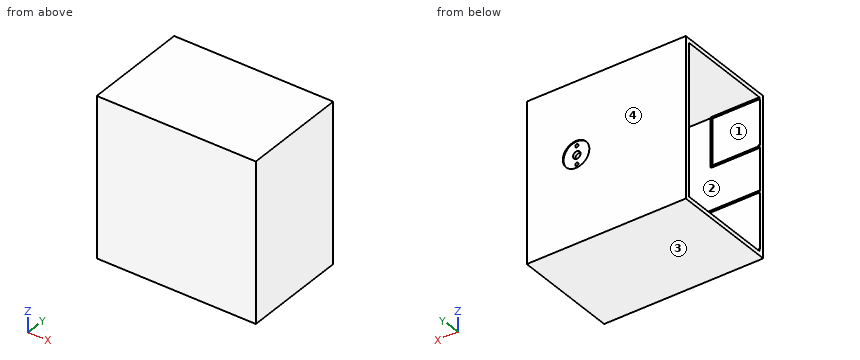
Autodesk Inventor part; units mm, degrees
ref_plane "YZ Plane" through (0, 0, 0) normal (1, 0, 0) x (0, 1, 0)
ref_plane "XZ Plane" through (0, 0, 0) normal (0, 1, 0) x (-1, 0, 0)
ref_plane "XY Plane" through (0, 0, 0) normal (0, 0, 1) x (1, 0, 0)
sketch "Boceto1" plane through (0, 0, 0) normal (0, 1, 0) x (-1, 0, 0)
  point P0 (0, 0)
extrude "Extrusión1" [suppressed]
feature "Vaciado1" [suppressed]
sketch "Boceto2" plane through (0, 70, 0) normal (0, 1, 0) x (1, 0, 0)
  line L0 (-5, 5) -> (-5, 145)
  line L1 (-145, 145) -> (-145, 5)
  line L2 (-145, 5) -> (-5, 5)
  line L3 (-5, 145) -> (-145, 145)
  line L4 (-150, 0) -> (0, 0)
  circle A0 centre (-46.4922, 78) radius 12.5
  circle A1 centre (-46.4922, 78) radius 13.5
hole "Agujero1" [suppressed]
sketch "Boceto3" plane through (0, 70, 0) normal (0, 1, 0) x (1, 0, 0)
  point P0 (0, 0)
sketch "Boceto4" plane through (0, 0, 0) normal (0, 1, 0) x (-1, 0, 0)
  point P0 (0, 0)
extrude "Extrusión2" [suppressed]
feature "Vaciado2" [suppressed]
sketch "Boceto5" plane through (0, 100, 0) normal (0, 1, 0) x (1, 0, 0)
  line L0 (0, 0) -> (0, 150)
  circle A0 centre (-46.5, 67.5) radius 14.5
extrude "Extrusión3" [suppressed]
sketch "Boceto6" plane through (0, 100, 0) normal (0, 1, 0) x (1, 0, 0)
  circle A0 centre (-46.5, 67.5) radius 12.5
extrude "Extrusión4" [suppressed]
sketch "Boceto7" plane through (-46.5, 31, -67.5) normal (0, -1, 0) x (1, 0, 0)
  point P0 (46.5, 67.5)
sketch "Boceto8" plane through (-46.5, 33, -67.5) normal (0, 1, 0) x (1, 0, 0)
  point P0 (46.5, -67.5)
sketch "Boceto9" plane through (0, 100, 0) normal (0, 1, 0) x (1, 0, 0)
  point P0 (0, 0)
sketch "Boceto10" plane through (0, 0, 0) normal (0, 1, 0) x (-1, 0, 0)
  line L0 (0, 0) -> (0, -150)
  line L1 (0, -150) -> (150, -150)
  line L2 (150, -150) -> (150, 0)
  line L3 (150, 0) -> (0, 0)
extrude "Extrusión5" add sketch "Boceto10" along normal blind 100
shell "Vaciado3" thickness 3 removed faces 1 at (-150, 33.3333, -100)
sketch "Boceto11" plane through (0, 100, 0) normal (0, 1, 0) x (1, 0, 0)
  line L0 (-150, 0) -> (0, 0)
  line L1 (0, 0) -> (0, 150)
  circle A0 centre (-46.5, 67.5) radius 12.5002
extrude "Extrusión6" add sketch "Boceto11" against normal blind 4
sketch "Boceto12" plane through (0, 100, 0) normal (0, 1, 0) x (1, 0, 0)
  circle A0 centre (-46.5, 67.5) radius 12.5
  point P0 (0, 0)
extrude "Extrusión7" cut sketch "Boceto12" against normal blind 1
sketch "Boceto13" plane through (0, 100, 0) normal (0, 1, 0) x (1, 0, 0)
  point P0 (0, 0)
sketch "Boceto14" plane through (-46.5, 96, -67.5) normal (0, -1, 0) x (1, 0, 0)
  circle A0 centre (0, 0) radius 3.5
  point P0 (46.5, 67.5)
extrude "Extrusión8" cut sketch "Boceto14" against normal blind 3
sketch "Boceto15" plane through (-46.5, 99, -67.5) normal (0, 1, 0) x (1, 0, 0)
  circle A0 centre (0, -8.5) radius 1.5
  circle A1 centre (0, 8.5) radius 1.5
  point P0 (46.5, -67.5)
extrude "Extrusión9" cut sketch "Boceto15" against normal blind 3
sketch "Boceto16" plane through (-150, 0, -150) normal (-1, 0, 0) x (0, 0, 1)
  line L0 (3, 97) -> (147, 97)
  line L1 (4, 96) -> (146, 96)
  line L2 (147, 3) -> (3, 3)
  line L3 (4, 4) -> (4, 96)
  line L4 (146, 4) -> (4, 4)
  line L5 (146, 96) -> (146, 4)
  line L6 (3, 97) -> (147, 97)
  line L7 (147, 3) -> (147, 97)
  line L8 (147, 3) -> (3, 3)
  line L9 (3, 3) -> (3, 97)
  line L10 (3, 97) -> (3, 3)
  line L11 (147, 97) -> (147, 3)
  point P0 (150, 0)
sketch "Boceto17" plane through (-150, 3, -147) normal (0, 0, 1) x (1, 0, 0)
  point P0 (150, -3)
extrude "Extrusión10" add sketch "Boceto16" against normal blind 148
sketch "Boceto18" plane through (-46.5, 97, -67.5) normal (0, 1, 0) x (1, 0, 0)
  circle A0 centre (0, 0) radius 3.5
  point P0 (46.5, -67.5)
extrude "Extrusión11" cut sketch "Boceto18" against normal blind 1
sketch "Boceto19" plane through (-150, 0, -150) normal (-1, 0, 0) x (0, 0, 1)
  point P0 (150, 0)
sketch "Boceto20" plane through (-46.5, 97, -76) normal (0, 1, 0) x (1, 0, 0)
  circle A0 centre (0, 0) radius 1.5
  circle A1 centre (0, 0) radius 1.5
  circle A2 centre (0, -17) radius 1.5
  point P0 (46.5, -76)
extrude "Extrusión12" cut sketch "Boceto20" against normal blind 1
sketch "Boceto21" plane through (-150, 0, -150) normal (-1, 0, 0) x (0, 0, 1)
  point P0 (150, 0)
sketch "Boceto22" plane through (-150, 4, -4) normal (0, 1, 0) x (1, 0, 0)
  point P0 (150, -4)
  point P1 (0, 142)
sketch "Boceto23" plane through (0, 0, 0) normal (0, -1, 0) x (1, 0, 0)
  point P0 (0, 0)
extrude "Extrusión13" [suppressed]
sketch "Boceto24" plane through (0, 5, 0) normal (0, 1, 0) x (1, 0, 0)
  point P0 (0, 0)
sketch "Boceto25" plane through (0, 0, 0) normal (0, -1, 0) x (1, 0, 0)
  line L0 (-150, -146) -> (-150, -4)
  line L1 (-150, -146) -> (-45.9, -146)
  line L2 (-45.9, -146) -> (-45.9, -90.1)
  line L3 (-45.9, -90.1) -> (-150, -90.1)
  line L4 (-150, -146) -> (-150, -145)
  line L5 (-149, -145) -> (-46.9, -145)
  line L6 (-45.9, -146) -> (-46.9, -146)
  line L7 (-46.9, -145) -> (-46.9, -91.1)
  line L8 (-45.9, -90.1) -> (-45.9, -91.1)
  line L9 (-46.9, -91.1) -> (-149, -91.1)
  line L10 (-150, -90.1) -> (-149, -90.1)
  line L11 (-149, -145) -> (-149, -144)
  line L12 (-149, -144) -> (-150, -144)
  line L13 (-149, -91.1) -> (-149, -92.1)
  line L14 (-149, -92.1) -> (-150, -92.1)
  line L15 (-149, -91.1) -> (-149, -92.1)
  line L16 (-149, -144) -> (-149, -145)
  line L17 (-150, -146) -> (-150, -144)
  line L18 (-150, -92.1) -> (-150, -90.1)
  point P0 (0, 0)
extrude "Extrusión14" add sketch "Boceto25" against normal blind 5 contours L0 L12 L11 L5 L7 L9 L13 L14 L3 L2 L1
sketch "Boceto26" plane through (-150, 4, -4) normal (0, 1, 0) x (1, 0, 0)
  line L0 (0, 0) -> (147, 0)
  line L1 (0, 0) -> (46, 0)
  line L2 (46, 0) -> (46, 46)
  line L3 (46, 46) -> (0, 46)
  line L4 (0, 0) -> (0, 86.1)
  line L5 (46, 46) -> (45, 46)
  line L6 (46, 46) -> (46, 45)
  line L7 (45, 45) -> (1, 45)
  line L8 (0, 46) -> (1, 46)
  line L9 (0, 0) -> (0, 1)
  line L10 (46, 46) -> (45, 46)
  line L11 (45, 45) -> (45, 1)
  line L12 (1, 1) -> (45, 1)
  line L13 (1, 45) -> (1, 44)
  line L14 (1, 44) -> (0, 44)
  line L15 (1, 1) -> (1, 2)
  line L16 (1, 2) -> (0, 2)
  line L17 (0, 46) -> (0, 44)
  line L18 (0, 2) -> (0, 0)
  line L19 (1, 45) -> (1, 44)
  line L20 (1, 2) -> (1, 1)
  point P0 (150, -4)
extrude "Extrusión15" add sketch "Boceto26" along normal blind 1 contours L4 L16 L15 L12 L11 L7 L13 L14 L3 L2 L0
properties part number "base"
Input: part model. Units: mm. Frame: model coordinates. Face numbers are marked on the shaded views. Coordinates: 2 decimals unless noted, no trailing zeros. Write each loop counter-clockwise with the first axis right and the second up, starting at its lowest first coordinate (ties: lowest second). Pieces come first, ordered by that corner, then holes. Notation, with made-up numbers: M 0.25,75 L 57.25,75 A26 ccw 57.25,91 Z; hole C -22.75,-28.75 d5. An arc over 180 degrees is marked long. Answer as a JSON object with one key per item and string values. Group by question number.
(1) Section A-A on x = -91.5. Output: boundary loops of the cut face in (y, z).
(2) Section C-C on y = 57.5. Output: boundary loops of the cut face in (x, z).
(3) Mould query, pull axis Z, two halves, no side actions, for the marked faces 1, 2, 3 and 4. Classes: pulls with the +Z half, pulls with the -Z half, needs draft (parallel to the pull), parting line crosses it, or undercut.
(4) Section B-B on z = -67.5. Output: boundary loops of the cut face in (x, y).
(5) Contact query for flat-ended pins moving along their axis: P1, Ø1.5, axis at y = 34, z = -84, coming from the +X side; P2, Ø8, axis at y = 27, z = -132, coming from the -X side; P3, Ø0.8, axis at y = 4.5, z = -131, coming from the -X side. Output: stop coordinate, or through.
(6) Ray query, line 1 along Z through (x, y) = (-46.5, 98.2); line 2 along Y through (x, z) = (-138.5, -127.5); line 3 along Z through (x, y) = (-134, 18). Return the intervals inside material, ascending. Write a range as [from, to].
(7) Section D-D on x = -15. Output: boundary loops of the cut face in (y, z).
Result set:
{
 "1": {"outline": "M 0,-150 L 100,-150 L 100,0 L 0,0 Z; hole M 4,-145 L 5,-145 L 5,-146 L 96,-146 L 96,-4 L 4,-4 L 4,-90.1 L 5,-90.1 L 5,-91.1 L 4,-91.1 Z"},
 "2": {"outline": "M -150,-150 L 0,-150 L 0,0 L -150,0 L -150,-4 L -3,-4 L -3,-146 L -150,-146 Z"},
 "3": {"face 1": "undercut", "face 2": "undercut", "face 3": "pulls with the -Z half", "face 4": "needs draft"},
 "4": {"outline": "M -150,0 L 0,0 L 0,100 L -34,100 L -34,99 L -43,99 L -43,96 L -3,96 L -3,4 L -150,4 Z; M -150,96 L -50,96 L -50,99 L -59,99 L -59,100 L -150,100 Z"},
 "5": {"P1": "stops at x = 0", "P2": "stops at x = -3", "P3": "stops at x = -46.9"},
 "6": {"line 1": "z = [-150, -77.5], [-74.5, -71], [-64, -60.5], [-57.5, 0]", "line 2": "y = [0, 4], [96, 100]", "line 3": "z = [-150, -146], [-4, 0]"},
 "7": {"outline": "M 0,-150 L 100,-150 L 100,0 L 0,0 Z; hole M 4,-146 L 96,-146 L 96,-4 L 4,-4 Z"}
}
